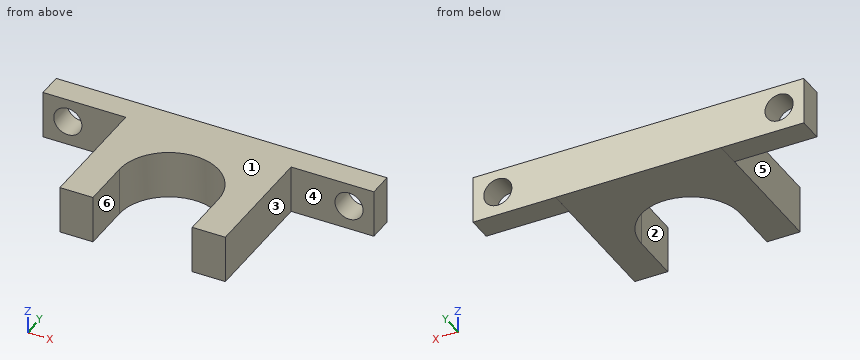
```python
from build123d import *

# Parameters (mm, degrees)
SKETCH091_W     = 20
SKETCH091_H     = 5.75
PAD030_DEPTH    = 18
POCKET028_DEPTH = 5.751
SKETCH093_W     = 10
SKETCH093_H     = 5.755
PAD031_DEPTH    = 3
SKETCH094_R     = 1.7
HOLE018_DEPTH   = 25


with BuildPart() as part:
    # Sketch091 → Pad030 (new body)
    with BuildSketch(Plane.XZ):
        with Locations((0, 208.435)):
            Rectangle(SKETCH091_W, SKETCH091_H)
    extrude(amount=PAD030_DEPTH)

    # Sketch092 (on Face4 of Pad030) → Pocket028 (cut, through all)
    with BuildSketch(Plane(origin=(0, 0, 211.31), x_dir=(-1, 0, 0), z_dir=(0, 0, 1))):
        with BuildLine():
            ThreePointArc((-6, 12), (0, 6), (6, 12))
            Line((6, 12), (6, 22))
            Line((-6, 22), (6, 22))
            Line((-6, 22), (-6, 12))
        make_face()
    extrude(amount=-POCKET028_DEPTH, mode=Mode.SUBTRACT)

    # Sketch093 → Pad031 (join)
    with BuildSketch(Plane.XZ):
        with Locations((-15, 208.4325)):
            Rectangle(SKETCH093_W, SKETCH093_H)
        with Locations((15, 208.4325)):
            Rectangle(SKETCH093_W, SKETCH093_H)
    extrude(amount=PAD031_DEPTH)

    # Sketch094 (on Face2 of Pad031) → Hole018 (cut)
    with BuildSketch(Plane.XZ.offset(3)):
        with Locations((-17, 208.5)):
            Circle(SKETCH094_R)
        with Locations((17, 208.5)):
            Circle(SKETCH094_R)
    extrude(amount=-HOLE018_DEPTH, mode=Mode.SUBTRACT)


with BuildPart() as part_1:
    # Body013 placement: moved
    add(part.part.moved(Location((0, 132, 0))))


solid = part_1.part
```
For this review, take the finished solid that the model builds, in its own axes (mm). Face numbers are marked on the shaded views. A direction names the side the tool comes from. Round coordinates to 2 decimals unless told otherwise and drop trailing zeros. Write each loop counter-clockwise with the first axis right and the second up, starting at its lowest first coordinate (ties: lowest second). Pieces come first, ordered by that corner, then holes. Notation, with made-up numbers: M 55.25,-33 L 63.25,-33 A27 ccw 63.25,-8 Z; hole C 42,65.5 d3. An arc over 180 degrees is marked long. One line per item, written item: value. Start each with the question number.
(1) We need section D-D (z = 206.15). Give the boundary of the cut face in (x, y), and give its area (3 significant figures).
(2) Wall thickness on line 1 (X direction, y = 131.3, z = 208.5); line 2 (Z direction, x = 17, y = 130.5) (3 decimals); line 3 (X direction, y = 129.25, z = 207.7): over which ranges is each line inside the solid? List them lowest first.
(3) We need section A-A (z = 208.5). Give the boundary of the cut face in (x, y), and give its area (3 significant figures).
(4) We need section C-C (y = 121.25). Give the boundary of the cut face in (x, z).
(5) Machinability: for the marked faces 4, 5 and 6, which of the approach directions +Z, -Z, +X, -X, +Y, -Y give a long, thin tool a straight path to every point of the face, cutting with its end or side? Answer none if there is none.
(6) Insertion check: pin 1 (3 mm diameter, centred on x = -12.5, z = 209, fed in from -Y); pin 2 (9 mm diameter, centred on x = -2, y = 126.5, fed in from -Z); pin 3 (2 mm diameter, centred on x = -4.5, y = 118, fed in from +Z); pin 4 (1 mm diameter, centred on y = 119.5, z = 210.5, fed in from -X). Each pin has a flat end and moves straight along its axis. Give the tip position at first contact, or say it passes through.
(7) We need section B-B (x = 17). Give the boundary of the cut face in (y, z) (3 decimals), and give its area (4 significant figures).
(8) The part is to be moulded in two halves that separate along X. For the marked faces 1, 2 and 3, say which applies: released by +X, released by -X, zero draft, split by the parting line, or undercut.
Result:
1. outline: M -20,129 L -10,129 L -10,114 L -6,114 L -6,120 A6 cw 6,120 L 6,114 L 10,114 L 10,129 L 20,129 L 20,132 L -20,132 Z
1. area: 291 mm²
2. line 1: -20 to -18.7, -15.3 to 15.3, 18.7 to 20
2. line 2: 205.555 to 206.8, 210.2 to 211.31
2. line 3: -20 to -18.5, -15.5 to 15.5, 18.5 to 20
3. outline: M -20,129 L -18.7,129 L -18.7,132 L -20,132 Z; M -15.3,129 L -10,129 L -10,114 L -6,114 L -6,120 A6 cw 6,120 L 6,114 L 10,114 L 10,129 L 15.3,129 L 15.3,132 L -15.3,132 Z; M 18.7,129 L 20,129 L 20,132 L 18.7,132 Z
3. area: 271 mm²
4. outline: M -10,205.56 L -5.87,205.56 L -5.87,211.31 L -10,211.31 Z; M 5.87,205.56 L 10,205.56 L 10,211.31 L 5.87,211.31 Z
5. face 4: +Z, -Z, +X, -Y
5. face 5: +Z, -Z, -X, -Y
5. face 6: +Z, -Z, -Y
6. pin 1: y = 129
6. pin 2: z = 205.56
6. pin 3: through
6. pin 4: x = -10
7. outline: M 129,205.555 L 132,205.555 L 132,206.8 L 129,206.8 Z; M 129,210.2 L 132,210.2 L 132,211.31 L 129,211.31 Z
7. area: 7.065 mm²
8. face 1: zero draft
8. face 2: undercut
8. face 3: released by +X
